The listing builds one solid part. Answer for the finished solid, in the listing's coordinates (mm). Face numbers are marked on the shaded views. A direction names the side the tool comes from. Coordinates: 2 decimals unless noted, no trailing zeros. Write each loop counter-clockwise with the first axis right and the second up, starting at its lowest first coordinate (ties: lowest second). Pieces come first, ordered by that corner, then holes.
(1) The part is cut by section B-B on z = -48.5. Determine the outline of the cut face in (x, y), plus the area to 3 significant figures.
(2) Straight lines are drawn through the part: line 1 (Y direction, x = -0.5, z = -105); line 2 (Z direction, x = -3.75, y = 4.25). For each, find the intervals that lie inside material, in ascending order.
(3) Given P1, Ø1.5, axis at x = -5, z = -78, coming from the +Y side; P2, Ø8, axis at y = -0.5, z = -104.5, coming from the -X side; P3, Ø1, axis at y = 5.5, z = -43.5, coming from the -X side, each flat-ended and moving along its own axis, determine where each tip first touches the part or whether it passes through.
(4) Which of the six approach directions +Z, -Z, +X, -X, +Y, -Y give full straight-line access (tool end or side, diameter ignored) to the marked faces 1 and 2?
(5) The part is cut by section A-A on z = -81.5. Determine the outline of the cut face in (x, y), plus the area to 3 significant figures.
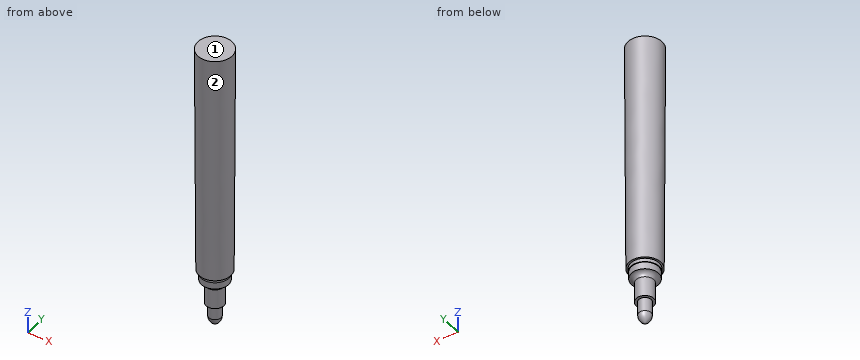
from build123d import *


with BuildPart() as part:
    # 草图1 → 旋转1 (revolve)
    with BuildSketch(Plane(origin=(0, 0, 0), x_dir=(1, 0, 0), z_dir=(0, 1, 0))):
        Polygon((0, 0), (-7.25, 0), (-6.75, 98.698733528), (0, 98.698733528), align=None)
    revolve(axis=Axis((0, 0, 0), (0, 0, 1)))

    # 草图2 → 旋转2 (revolve)
    with BuildSketch(Plane(origin=(0, 0, 0), x_dir=(1, 0, 0), z_dir=(0, 1, 0))):
        with BuildLine():
            Line((-6, 98.698733528), (-6, 100.198733528))
            Line((-6, 100.198733528), (-5.75, 100.198733528))
            Line((-5.75, 100.198733528), (-5.75, 103.198733528))
            ThreePointArc((-5.75, 103.198733528), (-4.335786438, 103.784519965), (-3.75, 105.198733528))
            Line((-3.75, 105.198733528), (-3.75, 113.598733528))
            Line((-3.75, 113.598733528), (-2.6, 113.598733528))
            Line((-2.6, 113.598733528), (-2.6, 119.451734729))
            ThreePointArc((-2.6, 119.451734729), (-1.886335345, 121.732085579), (0, 123.198733528))
            Line((0, 123.198733528), (0, 98.698733528))
            Line((0, 98.698733528), (-6, 98.698733528))
        make_face()
    revolve(axis=Axis((0, 0, -98.698733528), (0, 0, 1)))


solid = part.part
Model answer:
1. outline: circle Ø14.01 at (0, 0)
1. area: 154 mm2
2. line 1: y = -3.73 to 3.73
2. line 2: z = -103.2 to 0
3. P1: stops at y = 5.38
3. P2: stops at x = -5.75
3. P3: stops at x = -4.94
4. face 1: +Z, +X, -X, +Y, -Y
4. face 2: -Z
5. outline: circle Ø13.67 at (0, 0)
5. area: 147 mm2
